Input: dimensioned drawing with shaded views. Units: mm. Origin: part minimum x, y, z. Give positions to 0.01 mm unless a question says otherwise; leave off trailing zeros. Loops run counter-clockwise (first coordinate to the right, second up) from the corner with the lowest first, then second, coordinate; pieces in that order, holes last. Notation, with made-up numbers: (89.5, -30.5) -> (146.5, -30.5) arc R13 ccw to (146.5, -18.5) -> close; hole circle Ø3 at (80, 81). An arc over 180 degrees is marked (long way). One line per question, with ' | ' between items. Start each with the question number.
Item 1: Section D-D on x = 1. Return loops of the section in (y, z), then the cut area to 3 significant figures.
Item 2: Pin query (flat end, axial travel): P1, Ø3, axis at x = 3.5, z = 13, coming from the -Y side (1 decimal). Return the tip coordinate at first contact, or that it passes through.
Item 3: Section B-B on y = 2. Give the number of separate pieces and of enclosed holes in the cut face.
Item 4: Section C-C on x = 5.5. Return loops of the section in (y, z) (1 decimal), then the cut area to 3 significant figures.
Item 5: Material intervals for line 1 along Z through (x, y) = (6, 3.25) (1 decimal); line 2 along Z through (x, y) = (5.5, 8.5) (1 decimal); line 3 along Z through (x, y) = (4, 8), sorted ascending. Write a range as [from, to].
Item 6: Mould query, pull axis Z, two halves, no side actions, for the marked faces 1, 2 and 3. Classes: released by +Z, released by -Z, zero draft, split by the parting line, or undercut.
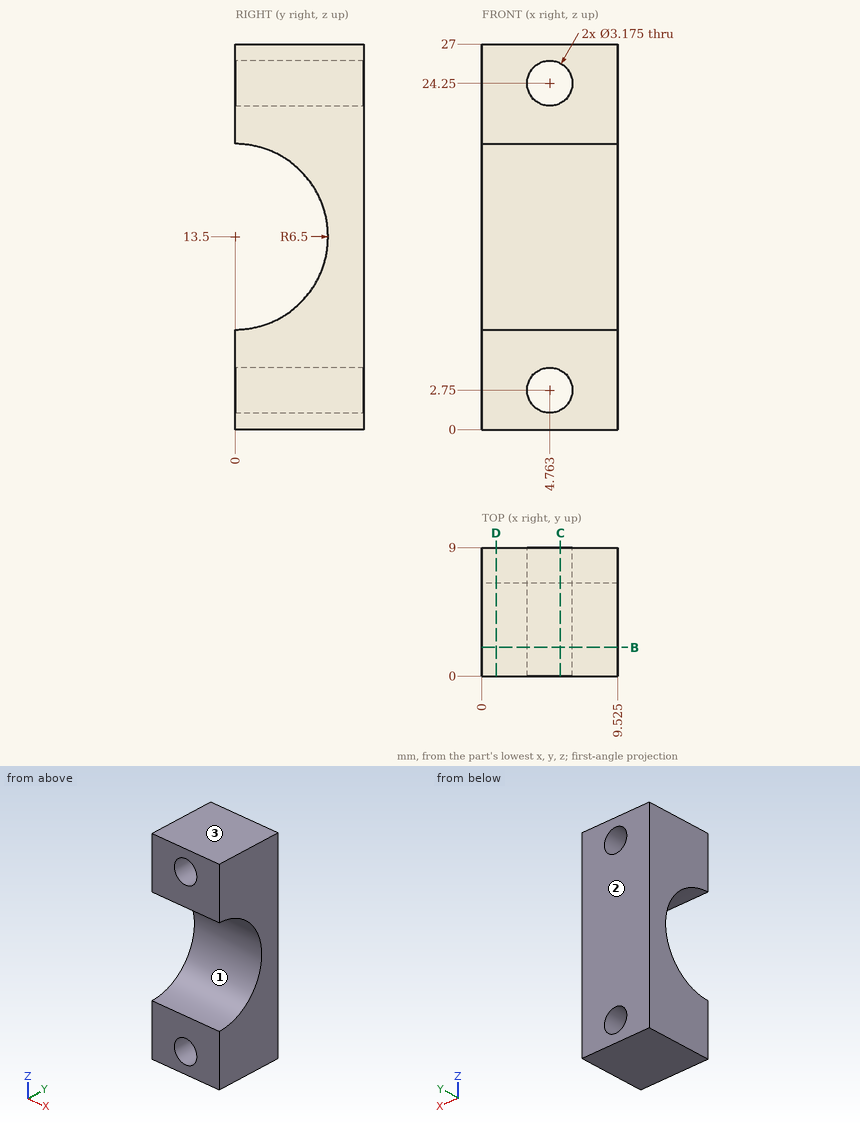
Result sheet:
1) outline: (0, 0) -> (9, 0) -> (9, 27) -> (0, 27) -> (0, 20) arc R6.5 cw to (0, 7) -> close | area: 177 mm²
2) P1: stops at y = 6.2
3) separate pieces: 2 | enclosed holes: 2
4) outline: (0, 0) -> (9, 0) -> (9, 1.3) -> (0, 1.3) -> close; (0, 4.2) -> (9, 4.2) -> (9, 22.8) -> (0, 22.8) -> (0, 20) arc R6.5 cw to (0, 7) -> close; (0, 25.7) -> (9, 25.7) -> (9, 27) -> (0, 27) -> close | area: 126 mm²
5) line 1: z = [0, 1.8], [3.7, 7.9], [19.1, 23.3], [25.2, 27] | line 2: z = [0, 1.3], [4.2, 22.8], [25.7, 27] | line 3: z = [0, 1.36], [4.14, 22.86], [25.64, 27]
6) face 1: undercut | face 2: zero draft | face 3: released by +Z
